Read the model definition and answer for the solid it produces. Units are mm, in the model's axes. Face numbers are marked on the shaded views. A direction names the side the tool comes from. Coordinates: 2 decimals unless noted, no trailing zeros. Write each loop counter-clockwise with the first axis right and the second up, starting at its lowest first coordinate (ties: lowest second). Pieces come first, ordered by that corner, then holes.
(1) Given pin 1 (18 mm diameter, centred on y = 29, z = 90.5, fed in from -X); pin 2 (3 mm diameter, centred on y = 18.5, z = 176, fed in from -X); pin 3 (8 mm diameter, centred on x = 165, z = 73.5, fed in from +Y), each flat-ended and moving along its own axis, determine where each tip first touches the part or whether it passes through.
(2) Section C-C on x = 29 is taken. Write down the section's boundary in (y, z), then the cut area to 3 significant figures.
(3) Which of the six approach directions +Z, -Z, +X, -X, +Y, -Y give full straight-line access (tool end or side, diameter ignored) to the marked faces 4, 5, 6 and 7?
(4) Section D-D on y = 79.5 is taken. Write down the section's boundary in (x, z), then the cut area to 3 significant figures.
(5) Section B-B on x = -4.5 is taken. Write down the section's boundary in (y, z).
(6) Find the intervals of material crossed by probe 1 along Y at (x, z) = (111, 59); probe 2 along X at (y, z) = (41, 94.5); probe 3 along Z at (x, y) = (244.5, 68.5), in increasing order.
(7) Section A-A on z = 40 is taken. Write down the section's boundary in (x, y).
(8) The mould has two halves that part along Z. Classify the marked faces 1, 2 and 3: +Z half, -Z half, draft (parallel to the pull), parting line (faces both ways), or undercut.
from build123d import *

# Parameters (mm, degrees)
SKETCH1_W                = 234
SKETCH1_H                = 66
SKETCH1_W_2              = 228
SKETCH1_H_2              = 60
BOSS_EXTRUDE1_DEPTH      = 243
BOSS_EXTRUDE2_DEPTH      = 66
SKETCH3_W                = 141
SKETCH3_H                = 60
SKETCH4_W                = 312
SKETCH4_H                = 24
BOSS_EXTRUDE3_DEPTH      = 147
BOSS_EXTRUDE3_DEPTH_BACK = 81


with BuildPart() as part:
    # Sketch1 → Boss-Extrude1 (new body)
    with BuildSketch(Plane.XY):
        with Locations((117, 33)):
            Rectangle(SKETCH1_W, SKETCH1_H)
        with Locations((117, 33)):
            Rectangle(SKETCH1_W_2, SKETCH1_H_2, mode=Mode.SUBTRACT)
    extrude(amount=BOSS_EXTRUDE1_DEPTH)

    # Sketch2 → Boss-Extrude2 (add)
    with BuildSketch(Plane.XZ):
        with BuildLine():
            Line((-27, 243), (261, 243))
            ThreePointArc((261, 243), (117, 99), (-27, 243))
        make_face()
    extrude(amount=-BOSS_EXTRUDE2_DEPTH)

    # Sketch3 → Cut-Revolve1 (revolve, cut)
    with BuildSketch(Plane.XY.offset(243)):
        with Locations((187.5, 33)):
            Rectangle(SKETCH3_W, SKETCH3_H)
    revolve(axis=Axis((117, 63, 243), (0, -1, 0)), mode=Mode.SUBTRACT)

    # Sketch4 → Boss-Extrude3 (add, two sides)
    with BuildSketch(Plane(origin=(0, 0, 0), x_dir=(1, 0, 0), z_dir=(0, 1, 0))) as boss_extrude3_sk:
        with Locations((117, 12)):
            Rectangle(SKETCH4_W, SKETCH4_H)
    extrude(amount=BOSS_EXTRUDE3_DEPTH)
    extrude(boss_extrude3_sk.sketch, amount=-BOSS_EXTRUDE3_DEPTH_BACK)


solid = part.part
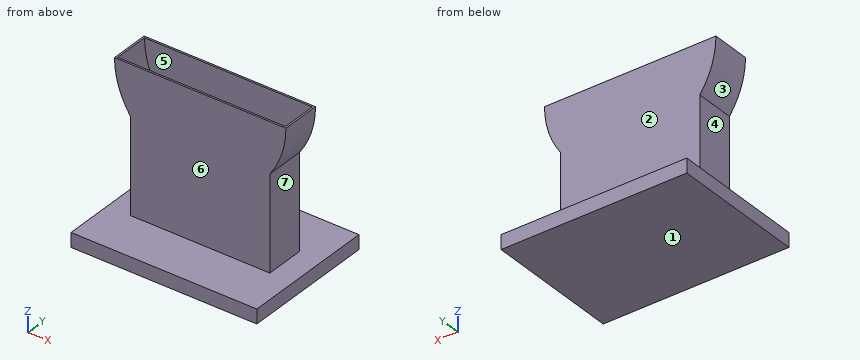
Response:
1. pin 1: stops at x = 0
1. pin 2: stops at x = -11.24
1. pin 3: stops at y = 66
2. outline: (-81, -24) - (147, -24) - (147, 0) - (66, 0) - (66, 243) - (63, 243) - (63, 132.83) - (3, 132.83) - (3, 243) - (0, 243) - (0, 0) - (-81, 0) - close; hole (3, 0) - (63, 0) - (63, 129.02) - (3, 129.02) - close
2. area: 7,160 mm2
3. face 4: -X, +Y, -Y
3. face 5: +Z
3. face 6: +Z, +X, -X, -Y
3. face 7: +X, +Y, -Y
4. outline: (-39, -24) - (273, -24) - (273, 0) - (-39, 0) - close
4. area: 7,490 mm2
5. outline: (-81, -24) - (147, -24) - (147, 0) - (-81, 0) - close; (0, 165.71) - (66, 165.71) - (66, 243) - (63, 243) - (63, 171.45) - (3, 171.45) - (3, 243) - (0, 243) - close
6. probe 1: y = 0 to 3, 63 to 66
6. probe 2: x = 0 to 3, 231 to 234
6. probe 3: z = -24 to 0
7. outline: (0, 0) - (234, 0) - (234, 66) - (0, 66) - close; hole (3, 3) - (231, 3) - (231, 63) - (3, 63) - close
8. face 1: -Z half
8. face 2: draft
8. face 3: undercut
